Here's how the part is built. I have some questions about the finished solid (model axes, mm). A direction names the side the tool comes from. Round coordinates to 2 decimals unless told otherwise and drop trailing zeros. Order: outer loops, then holes, each group sorted by start corner. A loop starts at its lowest first (then second) coordinate and runs counter-clockwise, first axis right, second up. Notation, with made-up numbers: (31.25, 80.25) - (43.25, 80.25) arc R26 cw to (43.25, 99.25) - close; hole circle Ø3 at (57.25, 9.25). An arc over 180 degrees is marked (long way). One line per item, written item: value.
from build123d import *

# Parameters (mm, degrees)
BASE_EXTRUDE_DEPTH                             = 3
BASE_START                                     = -3
BASE_CENTER_FILL_DEPTH                         = 3
HYDRA_CRADDLE_INSERT_DEPTH                     = 3
WEIGHT_RELIEF_DEPTH                            = 46.043730576
WEIGHT_RELIEF_DEPTH_BACK                       = 46.043730576
SKETCH6_R                                      = 1.25
SCREWHOLES_TO_HYDRA_CRADDLE_DEPTH              = 10
FILLET1_R                                      = 10
FILLET2_R                                      = 5
SPACER_BETWEEN_HYDRA_STACK_AND_E_MATCH_C_DEPTH = 3
EMATCH_WIRE_CLEARANCE_CUT_DEPTH                = 46.540505752
EMATCH_WIRE_CLEARANCE_CUT_DEPTH_BACK           = 3
SKETCH9_W                                      = 20
SKETCH9_H                                      = 5
ALIGNMENT_PEG_WITH_BLAST_SHIELD_DEPTH          = 5
FILLET3_R                                      = 1
FILLET4_R                                      = 0.5


with BuildPart() as part:
    # Sketch1 → BASE EXTRUDE (new body)
    with BuildSketch(Plane.XY.offset(25)):
        with BuildLine():
            Line((0, 19.861263432), (6, 19.861263432))
            Line((6, 19.861263432), (6, 24))
            ThreePointArc((6, 24), (6.4, 24.8), (7.28, 24.96))
            ThreePointArc((7.28, 24.96), (25.292757683, 6.022990019), (17.748239349, -19))
            Line((17.748239349, -19), (19.902899824, -19))
            ThreePointArc((19.902899824, -19), (21.19699505, -19.170370869), (22.402899824, -19.669872981))
            Line((22.402899824, -19.669872981), (24.772193743, -21.037785463))
            ThreePointArc((24.772193743, -21.037785463), (28.145825623, -16.25), (30.605353521, -10.934456357))
            Line((30.605353521, -10.934456357), (30.369621377, -10.79835634))
            ThreePointArc((30.369621377, -10.79835634), (28.317417482, -8.536426532), (27.963707738, -5.50282196))
            ThreePointArc((27.963707738, -5.50282196), (24.719171834, 14.184940742), (9.358208955, 26.919768297))
            ThreePointArc((9.358208955, 26.919768297), (6.925140786, 28.74503188), (6, 31.642534665))
            Line((6, 31.642534665), (6, 31.941352507))
            ThreePointArc((6, 31.941352507), (3.012975565, 32.360036747), (0, 32.5))
            ThreePointArc((0, 32.5), (-3.012975565, 32.360036747), (-6, 31.941352507))
            Line((-6, 31.941352507), (-6, 31.642534665))
            ThreePointArc((-6, 31.642534665), (-6.925140786, 28.74503188), (-9.358208955, 26.919768297))
            ThreePointArc((-9.358208955, 26.919768297), (-24.719171834, 14.184940742), (-27.963707738, -5.50282196))
            ThreePointArc((-27.963707738, -5.50282196), (-28.317417482, -8.536426532), (-30.369621377, -10.79835634))
            Line((-30.369621377, -10.79835634), (-30.605353521, -10.934456357))
            ThreePointArc((-30.605353521, -10.934456357), (-28.145825623, -16.25), (-24.772193743, -21.037785463))
            Line((-24.772193743, -21.037785463), (-22.402899824, -19.669872981))
            ThreePointArc((-22.402899824, -19.669872981), (-21.19699505, -19.170370869), (-19.902899824, -19))
            Line((-19.902899824, -19), (-17.748239349, -19))
            ThreePointArc((-17.748239349, -19), (-25.292757683, 6.022990019), (-7.28, 24.96))
            ThreePointArc((-7.28, 24.96), (-6.4, 24.8), (-6, 24))
            Line((-6, 24), (-6, 19.861263432))
            Line((-6, 19.861263432), (0, 19.861263432))
        make_face()
    extrude(amount=BASE_EXTRUDE_DEPTH)

    # Sketch3 → BASE CENTER FILL (add)
    with BuildSketch(Plane.XY.offset(28).offset(BASE_START)):
        with BuildLine():
            Line((-17.748239349, -19), (17.748239349, -19))
            ThreePointArc((17.748239349, -19), (0, 26), (-17.748239349, -19))
        make_face()
    extrude(amount=BASE_CENTER_FILL_DEPTH)

    # Sketch4 → HYDRA CRADDLE INSERT (add)
    with BuildSketch(Plane(origin=(0, 0, 25), x_dir=(-1, 0, 0), z_dir=(0, 0, -1))):
        with BuildLine():
            Line((-6.25, 23.763154252), (-9.25, 23.763154252))
            ThreePointArc((-9.25, 23.763154252), (-25.090515447, 4.551487076), (-17.007351352, -19))
            Line((-17.007351352, -19), (17.007351352, -19))
            ThreePointArc((17.007351352, -19), (25.090515447, 4.551487076), (9.25, 23.763154252))
            Line((9.25, 23.763154252), (6.25, 23.763154252))
            Line((6.25, 23.763154252), (6.25, 19.5))
            Line((6.25, 19.5), (-6.25, 19.5))
            Line((-6.25, 19.5), (-6.25, 23.763154252))
        make_face()
    extrude(amount=HYDRA_CRADDLE_INSERT_DEPTH)

    # Sketch5 → WEIGHT RELIEF (cut, two sides: drawn at the far end of the back side and taken through both)
    with BuildSketch(Plane(origin=(0, 0, 22), x_dir=(-1, 0, 0), z_dir=(0, 0, -1)).offset(-WEIGHT_RELIEF_DEPTH_BACK)):
        with BuildLine():
            Line((-14.142135624, 17.5), (14.142135624, 17.5))
            ThreePointArc((14.142135624, 17.5), (22.471855433, 1.125039286), (15.81929202, -16))
            Line((15.81929202, -16), (-15.81929202, -16))
            ThreePointArc((-15.81929202, -16), (-22.471855433, 1.125039286), (-14.142135624, 17.5))
        make_face()
    extrude(amount=WEIGHT_RELIEF_DEPTH + WEIGHT_RELIEF_DEPTH_BACK, mode=Mode.SUBTRACT)

    # Sketch6 → SCREWHOLES TO HYDRA CRADDLE (cut)
    with BuildSketch(Plane(origin=(0, 0, 25), x_dir=(-1, 0, 0), z_dir=(0, 0, -1))):
        with Locations((-25.547749412, -14.75)):
            Circle(SKETCH6_R)
        with Locations((25.547749412, -14.75)):
            Circle(SKETCH6_R)
        with Locations((-3, 29.5)):
            Circle(SKETCH6_R)
        with Locations((3, 29.5)):
            Circle(SKETCH6_R)
    extrude(amount=-SCREWHOLES_TO_HYDRA_CRADDLE_DEPTH, mode=Mode.SUBTRACT)

    # Fillet1
    fillet1_edges = [part.edges().sort_by_distance(p)[0] for p in [
        (15.81929202, -16, 25),
        (-15.81929202, -16, 25),
    ]]
    fillet(fillet1_edges, radius=FILLET1_R)

    # Fillet2
    fillet2_edges = [part.edges().sort_by_distance(p)[0] for p in [
        (14.142135624, 17.5, 25),
        (-14.142135624, 17.5, 25),
    ]]
    fillet(fillet2_edges, radius=FILLET2_R)

    # Sketch7 → SPACER BETWEEN HYDRA STACK AND E-MATCH CRADDLES (add)
    with BuildSketch(Plane.XY.offset(28)):
        with BuildLine():
            Line((-9.358208955, 26.919768297), (9.358208955, 26.919768297))
            ThreePointArc((9.358208955, 26.919768297), (24.719171834, 14.184940742), (27.963707738, -5.50282196))
            Line((27.963707738, -5.50282196), (19.902899824, -19))
            Line((19.902899824, -19), (-19.902899824, -19))
            Line((-19.902899824, -19), (-27.963707738, -5.50282196))
            ThreePointArc((-27.963707738, -5.50282196), (-24.719171834, 14.184940742), (-9.358208955, 26.919768297))
        make_face()
        with BuildLine():
            Line((10.9658561, -16), (-10.9658561, -16))
            ThreePointArc((-10.9658561, -16), (-16.064875613, -14.602325267), (-19.73854098, -10.8))
            ThreePointArc((-19.73854098, -10.8), (-22.255771186, 3.306153192), (-15.746719775, 16.071428571))
            ThreePointArc((-15.746719775, 16.071428571), (-14.137271079, 17.129100499), (-12.247448714, 17.5))
            Line((-12.247448714, 17.5), (12.247448714, 17.5))
            ThreePointArc((12.247448714, 17.5), (14.137271079, 17.129100499), (15.746719775, 16.071428571))
            ThreePointArc((15.746719775, 16.071428571), (22.255771186, 3.306153192), (19.73854098, -10.8))
            ThreePointArc((19.73854098, -10.8), (16.064875613, -14.602325267), (10.9658561, -16))
        make_face(mode=Mode.SUBTRACT)
    extrude(amount=SPACER_BETWEEN_HYDRA_STACK_AND_E_MATCH_C_DEPTH)

    # Sketch8 → EMATCH WIRE CLEARANCE CUT (cut, two sides: drawn at the far end of the back side and taken through both)
    with BuildSketch(Plane.XY.offset(31).offset(-EMATCH_WIRE_CLEARANCE_CUT_DEPTH_BACK)):
        with BuildLine():
            Line((-17.492855685, 22.5), (17.492855685, 22.5))
            ThreePointArc((17.492855685, 22.5), (13.606193664, 25.042393935), (9.358208955, 26.919768297))
            Line((9.358208955, 26.919768297), (-9.358208955, 26.919768297))
            ThreePointArc((-9.358208955, 26.919768297), (-13.606193664, 25.042393935), (-17.492855685, 22.5))
        make_face()
    extrude(amount=EMATCH_WIRE_CLEARANCE_CUT_DEPTH + EMATCH_WIRE_CLEARANCE_CUT_DEPTH_BACK, mode=Mode.SUBTRACT)

    # Sketch9 → ALIGNMENT PEG WITH BLAST SHIELD (add)
    with BuildSketch(Plane.XY.offset(31)):
        with Locations((0, 20)):
            Rectangle(SKETCH9_W, SKETCH9_H)
    extrude(amount=ALIGNMENT_PEG_WITH_BLAST_SHIELD_DEPTH)

    # Fillet3
    fillet3_edges = [part.edges().sort_by_distance(p)[0] for p in [
        (0, 22.5, 28),
        (-10, 20, 31),
        (10, 20, 31),
    ]]
    fillet(fillet3_edges, radius=FILLET3_R)

    # Fillet4
    fillet4_edges = [part.edges().sort_by_distance(p)[0] for p in [
        (7.75, 23.763154252, 22),
        (6.25, 23.763154252, 23.5),
        (25.090515447, 4.551487076, 25),
        (9.25, 23.763154252, 23.5),
        (-25.090515447, 4.551487076, 25),
        (-7.75, 23.763154252, 22),
        (-9.25, 23.763154252, 23.5),
        (-6.25, 21.631577126, 22),
        (-6.25, 23.763154252, 23.5),
        (0, 19.5, 22),
        (6.25, 21.631577126, 22),
        (6.25, 19.5, 23.5),
        (25.090515447, 4.551487076, 22),
        (0, -19, 22),
        (-25.090515447, 4.551487076, 22),
        (7.75, 23.763154252, 25),
        (6.25, 21.631577126, 25),
        (0, 19.5, 25),
        (-6.25, 21.631577126, 25),
        (-7.75, 23.763154252, 25),
        (-22.255771186, 3.306153192, 22),
        (0, -16, 22),
        (-16.064875613, -14.602325267, 22),
        (16.064875613, -14.602325267, 22),
        (0, 17.5, 22),
        (22.255771186, 3.306153192, 22),
        (-14.137271079, 17.129100499, 22),
        (14.137271079, 17.129100499, 22),
    ]]
    fillet(fillet4_edges, radius=FILLET4_R)


solid = part.part
Q1. We'd pull the mould along X, two halves only. Please class faces 4 (the flat face through (-23.877, -12.346, 29.479)), 5 (the cylindrical face through (28.105, -16.321, 26.479)), 6 (the flat face through (-6.25, 21, 24)): released by +X, released by -X, zero draft, split by the parting line, or undercut.
Results list:
face 4: released by -X
face 5: released by +X
face 6: undercut
Q2. Will these pins go through, and if not, where does the flat tip stop? pin 1 (3 mm diameter, centred on y = 19, z = 33.5, fed in from +X); pin 2 (1.6 mm diameter, centred on y = 21, z = 23.5, fed in from +X); pin 3 (5 mm diameter, centred on x = -6.5, z = 24, fed in from -Y).
Results list:
pin 1: x = 10
pin 2: x = 15.56
pin 3: y = -19
Q3. Which directions (+Z, -Z, +X, -X, +Y, -Y) give clear straight access to the entire face, cutting with the end or side of a thin tool? Please do faces 1 (the flat face through (10, 20, 34)), 2 (the cylindrical face through (-21.215, -19.175, 26.479)), 3 (the cylindrical face through (-25.16, 4.15, 23.51)).
Results list:
face 1: +Z, +X, +Y, -Y
face 2: +Z, -Z, -Y
face 3: -Z, -X
Q4. If we section it at D-D, the plane z = 34.75: Please give me the cut outline in (x, y).
Results list:
outline: (-10, 17.5) - (10, 17.5) - (10, 22.5) - (-10, 22.5) - close
Q5. If we section it at C-C, the plane x = 3: Please give me the cut outline in (y, z), then the cut area to 3 significant figures.
Results list:
outline: (-19, 22.5) arc R0.5 ccw to (-18.5, 22) - (-16.5, 22) arc R0.5 ccw to (-16, 22.5) - (-16, 31) - (-19, 31) - close; (17.5, 22.5) arc R0.5 ccw to (18, 22) - (19, 22) arc R0.5 ccw to (19.5, 22.5) - (19.5, 24.5) arc R0.5 cw to (20, 25) - (28.25, 25) - (28.25, 28) - (23.5, 28) arc R1 cw to (22.5, 29) - (22.5, 36) - (17.5, 36) - close; (30.75, 25) - (32.36, 25) - (32.36, 28) - (30.75, 28) - close
area: 110 mm²
Q6. If I drill on line 1 along Z through (x, y) = (23.5, 5); line 2 along Y through (x, z) = (3, 26.8); line 3 along X through (y, z) = (17, 26), over which ranges is the centre line in solid material (lowest first)?
Results list:
line 1: 22 to 31
line 2: -19 to -16, 17.5 to 28.25, 30.75 to 32.36
line 3: -22.87 to -14.43, 14.43 to 22.87
Q7. If we section it at A-A, the plane y = 29.5: Please give me the cut outline in (x, z).
Results list:
outline: (-6.48, 25) - (-4.25, 25) - (-4.25, 28) - (-6.48, 28) - close; (-1.75, 25) - (1.75, 25) - (1.75, 28) - (-1.75, 28) - close; (4.25, 25) - (6.48, 25) - (6.48, 28) - (4.25, 28) - close
Q8. If we section it at B-B, the plane z = 26.5: Give the number of separate pieces and of enclosed holes in the cut face, then the cut area to 3 significant figures.
Results list:
separate pieces: 1
enclosed holes: 5
area: 1,060 mm²
